```python
from build123d import *

# Parameters (mm, degrees)
SKETCH_1_R          = 2.1
EXTRUDE_1_DEPTH     = 3
FILLET_1_R          = 10
SKETCH_2_R          = 3.1
CUT_EXTRUDE_1_DEPTH = 10
FILLET_2_R          = 10


with BuildPart() as part:
    # 草图1 → 凸台-拉伸1 (new body)
    with BuildSketch(Plane(origin=(0, 0, 0), x_dir=(1, 0, 0), z_dir=(0, 1, 0))):
        Polygon((-7.5, 55), (-7.5, -5), (42.5, -5), (42.5, 55), (42.5, 95), (12.189110868, 112.5), (-18.121778265, 130), (-70.083302492, 160), (-154.724318643, 160), (-189.365334795, 160), align=None)
        with Locations(Location((0, 0, 0), (0, 0, 270))):
            Circle(SKETCH_1_R, mode=Mode.SUBTRACT)
        with Locations(Location((35, 0, 0), (0, 0, 270))):
            Circle(SKETCH_1_R, mode=Mode.SUBTRACT)
        with Locations(Location((0, 50, 0), (0, 0, 270))):
            Circle(SKETCH_1_R, mode=Mode.SUBTRACT)
        with Locations(Location((35, 50, 0), (0, 0, 270))):
            Circle(SKETCH_1_R, mode=Mode.SUBTRACT)
    extrude(amount=EXTRUDE_1_DEPTH)

    # 圆角1
    fillet_1_edges = [part.edges().sort_by_distance(p)[0] for p in [
        (-70.083302492, 1.5, -160),
        (42.5, 1.5, -95),
        (-7.5, 1.5, -55),
        (-189.365334795, 1.5, -160),
    ]]
    fillet(fillet_1_edges, radius=FILLET_1_R)

    # 草图2 → 切除-拉伸1 (cut)
    with BuildSketch(Plane(origin=(0, 3, 0), x_dir=(1, 0, 0), z_dir=(0, 1, 0))):
        with Locations(Location((-152.37976321, 149.419872981, 0), (0, 0, 270))):
            Circle(SKETCH_2_R)
    extrude(amount=-CUT_EXTRUDE_1_DEPTH, mode=Mode.SUBTRACT)

    # 圆角2
    fillet_2_edges = [part.edges().sort_by_distance(p)[0] for p in [
        (42.5, 1.5, 5),
        (-7.5, 1.5, 5),
    ]]
    fillet(fillet_2_edges, radius=FILLET_2_R)


solid = part.part
```
Source: CAD feature listing. Evaluate the final solid. Frame: model axes, mm. Coordinates: 2 decimals unless noted, no trailing zeros. Write each loop counter-clockwise with the first axis right and the second up, starting at its lowest first coordinate (ties: lowest second). Pieces come first, ordered by that corner, then holes. Notation, with made-up numbers: (55.5, -1) -> (102.5, -1) arc R19 cw to (102.5, 30) -> close; hole circle Ø10 at (-28.75, 34.5). An arc over 180 degrees is marked (long way). Return JSON: item names as keys, results as strings. Group by question number.
1) Section query B-B, the plane x = 25.5. Return loops of the section in (y, z), plus the area to 3 significant figures.
2) Ray query, line 1 along X through (y, z) = (1.3, -50); line 2 along X through (y, z) = (2.3, 0); line 3 along X through (y, z) = (0.8, -114). Return the intervals inside material, ascending.
3) Mould query, pull axis Z, two halves, no side actions, for faces 1 (the face through (32.95, 1.48, -0.46)), 2 (the face through (-4.65, 1.52, 1.99)), 3 (the face through (33.137, 1.479, -49.031)), 4 (the face through (-38, 0, -97)). Classes: +Z half, -Z half, draft (parallel to the pull), parting line (faces both ways), or undercut.
4) Contact query for flat-ended pins moving along their axis: P1, Ø10, axis at x = -152.38, z = -149.42, coming from the -Y side; P2, Ø1.5, axis at y = 1, z = -26.5, coming from the -X side; P3, Ø1, axis at y = 1, z = -60, coming from the -X side. Output: stop coordinate, or through.
5) Section query A-A, the plane y = 2.5. Return loops of the section in (x, z), plus the area to 3 significant figures.
6) Section query C-C, the plane z = -23.5. Return loops of the section in (x, y), plus the area to 3 significant figures.
From the geometry:
{
 "1": {"outline": "(0, -104.81) -> (3, -104.81) -> (3, 5) -> (0, 5) -> close", "area": "329 mm²"},
 "2": {"line 1": "-7.53 to -2.1, 2.1 to 32.9, 37.1 to 42.5", "line 2": "-6.16 to -2.1, 2.1 to 32.9, 37.1 to 41.16", "line 3": "-109.69 to 9.59"},
 "3": {"face 1": "undercut", "face 2": "+Z half", "face 3": "undercut", "face 4": "draft"},
 "4": {"P1": "y = 0", "P2": "x = -7.5", "P3": "x = -17.03"},
 "5": {"outline": "(-157.04, -141.34) arc R10 ccw to (-152.04, -160) -> (-72.76, -160) arc R10 ccw to (-67.76, -158.66) -> (37.5, -97.89) arc R10 ccw to (42.5, -89.23) -> (42.5, -5) arc R10 ccw to (32.5, 5) -> (2.5, 5) arc R10 ccw to (-7.5, -5) -> (-7.5, -49.23) arc R10 cw to (-12.5, -57.89) -> close; hole circle Ø6.2 at (-152.38, -149.42); hole circle Ø4.2 at (0, -50); hole circle Ø4.2 at (0, 0); hole circle Ø4.2 at (35, -50); hole circle Ø4.2 at (35, 0)", "area": "13,800 mm²"},
 "6": {"outline": "(-7.5, 0) -> (42.5, 0) -> (42.5, 3) -> (-7.5, 3) -> close", "area": "150 mm²"}
}
